Part model, mm, in its own coordinate system. A direction names the side the tool comes from. Give positions to 0.01 mm unless a question says otherwise; leave off trailing zeros. Order: outer loops, then holes, each group sorted by start corner. A loop starts at its lowest first (then second) coordinate and runs counter-clockwise, first axis right, second up. Notation, with made-up numbers: (-13.75, 77.5) -> (24.25, 77.5) arc R22 ccw to (24.25, 94.5) -> close; hole circle Ø6 at (-31, 84). An arc over 180 degrees is marked (long way). Write item = value, one per line. Start each with the question number.
Item 1: Drill centre lines: line 1 along Y through (x, z) = (0, 0.8); line 2 along Y through (x, z) = (-1.25, -0.85); line 3 along Z through (x, y) = (0.75, -12.5). Where is each one in solid material? Low to high.
Item 2: Band-saw the part on D-D on x = -1.5. Write the cut outline in (y, z), plus the area to 3 significant figures.
Item 3: Band-saw the part on C-C on z = 1.8. Write the cut outline in (x, y), plus the area to 3 significant figures.
Item 4: Band-saw the part on B-B on y = -11.5. Write the cut outline in (x, z).
Item 5: Tool access for faces 4 (the face through (0, 14.5, 1)), 5 (the face through (-1, -10, 0)), 6 (the face through (-0.9, 10.6, 0)): list every direction of +Z, -Z, +X, -X, +Y, -Y with a clear straight run to the whole face (end or side of a thin tool).
Item 6: Flat gauge pins, fed straight in: P1, Ø3, axis at x = 1, y = 12.5, coming from the -Z side; P2, Ø1.6, axis at x = -1.5, z = -1, coming from the +Y side; P3, Ø1.8, axis at x = 0, y = 11.5, coming from the +Z side; P4, Ø0.6, axis at x = 0, z = -1, coming from the -Y side. Where does each tip first touch, or does it go through?
Item 7: Pull direction Y, two halves, no side cores. Call faces 1 (the face through (0, -14.5, 1)), 2 (the face through (0, 0, -2)), 3 (the face through (-0.238, -12.574, 1.521)): +Y half, -Y half, draft (parallel to the pull), parting line (faces both ways), or undercut.
Item 8: Band-saw the part on A-A on x = 0. Write the cut outline in (y, z), plus the area to 3 significant figures.
```python
from build123d import *

# Parameters (mm, degrees)
SKETCH_1_W            = 8
SKETCH_1_H            = 29
EXTRUDE_241_DEPTH     = 3
SKETCH_2_W            = 8
SKETCH_2_H            = 16
EXTRUDE_361_DEPTH     = 2
CUT_EXTRUDE_555_REACH = 17.851
SKETCH_3_R            = 1.1


with BuildPart() as part:
    # 草图1 → Extrude 241 (new body)
    with BuildSketch(Plane.XY):
        Rectangle(SKETCH_1_W, SKETCH_1_H)
    extrude(amount=EXTRUDE_241_DEPTH)

    # 草图2 → Extrude 361 (add)
    with BuildSketch(Plane.XY):
        Rectangle(SKETCH_2_W, SKETCH_2_H)
    extrude(amount=-EXTRUDE_361_DEPTH)

    # 草图3 → Cut-Extrude 555 (cut, up to next)
    with BuildSketch(Plane.XY.offset(3), mode=Mode.PRIVATE) as cut_extrude_555_sk1:
        with Locations((0, 11.5)):
            Circle(SKETCH_3_R)
    cut_extrude_555_tool1 = extrude(cut_extrude_555_sk1.sketch, amount=-CUT_EXTRUDE_555_REACH, mode=Mode.PRIVATE) & part.part
    # 草图3 → Cut-Extrude 555 (cut, up to next)
    with BuildSketch(Plane.XY.offset(3), mode=Mode.PRIVATE) as cut_extrude_555_sk2:
        with Locations((0, -11.5)):
            Circle(SKETCH_3_R)
    cut_extrude_555_tool2 = extrude(cut_extrude_555_sk2.sketch, amount=-CUT_EXTRUDE_555_REACH, mode=Mode.PRIVATE) & part.part
    add(cut_extrude_555_tool1.solids().sort_by_distance((0, 11.5, 3))[0], mode=Mode.SUBTRACT)
    add(cut_extrude_555_tool2.solids().sort_by_distance((0, -11.5, 3))[0], mode=Mode.SUBTRACT)


solid = part.part
```
Values found:
q1.line_1 = -14.5 to -12.6, -10.4 to 10.4, 12.6 to 14.5
q1.line_2 = -8 to 8
q1.line_3 = 0 to 3
q2.outline = (-14.5, 0) -> (-8, 0) -> (-8, -2) -> (8, -2) -> (8, 0) -> (14.5, 0) -> (14.5, 3) -> (-14.5, 3) -> close
q2.area = 119 mm^2
q3.outline = (-4, -14.5) -> (4, -14.5) -> (4, 14.5) -> (-4, 14.5) -> close; hole circle Ø2.2 at (0, -11.5); hole circle Ø2.2 at (0, 11.5)
q3.area = 224 mm^2
q4.outline = (-4, 0) -> (-1.1, 0) -> (-1.1, 3) -> (-4, 3) -> close; (1.1, 0) -> (4, 0) -> (4, 3) -> (1.1, 3) -> close
q5.face_4 = +Z, -Z, +X, -X, +Y
q5.face_5 = -Z, +X, -X, -Y
q5.face_6 = -Z, +X, -X, +Y
q6.P1 = 0
q6.P2 = 8
q6.P3 = through
q6.P4 = -8
q7.face_1 = -Y half
q7.face_2 = draft
q7.face_3 = undercut
q8.outline = (-14.5, 0) -> (-12.6, 0) -> (-12.6, 3) -> (-14.5, 3) -> close; (-10.4, 0) -> (-8, 0) -> (-8, -2) -> (8, -2) -> (8, 0) -> (10.4, 0) -> (10.4, 3) -> (-10.4, 3) -> close; (12.6, 0) -> (14.5, 0) -> (14.5, 3) -> (12.6, 3) -> close
q8.area = 106 mm^2
